Model file for the job. Use its own axes, mm. A direction names the side the tool comes from. Round coordinates to 2 decimals unless told otherwise and drop trailing zeros. Order: outer loops, then holes, each group sorted by start corner. A loop starts at its lowest first (then second) coordinate and runs counter-clockwise, first axis right, second up. Notation, with made-up numbers: (-1.75, 30) - (47.25, 30) arc R28 cw to (47.25, 64) - close; hole circle Ø4 at (27, -29). An arc over 180 degrees is marked (long way). Use one line per item in the form item = value.
from build123d import *

# Parameters (mm, degrees)
BOSS_EXTRUDE3_DEPTH = 59
SKETCH4_W           = 59
SKETCH4_H           = 59
BOSS_EXTRUDE4_DEPTH = 100
SHELL2_T            = -3
SKETCH5_W           = 59
SKETCH5_H           = 59
CUT_EXTRUDE1_DEPTH  = 100
FILLET1_R           = 10


with BuildPart() as part:
    # Sketch3 → Boss-Extrude3 (new body)
    with BuildSketch(Plane.XY):
        with BuildLine():
            Line((-32.434933876, -26.188574195), (26.565066124, -26.188574195))
            Line((26.565066124, -26.188574195), (26.565066124, -36.188574195))
            ThreePointArc((26.565066124, -36.188574195), (33.887396594, -53.866243725), (51.565066124, -61.188574195))
            Line((51.565066124, -61.188574195), (61.565066124, -61.188574195))
            Line((61.565066124, -61.188574195), (61.565066124, -120.188574195))
            Line((61.565066124, -120.188574195), (51.565066124, -120.188574195))
            ThreePointArc((51.565066124, -120.188574195), (-7.831903496, -95.585543815), (-32.434933876, -36.188574195))
            Line((-32.434933876, -36.188574195), (-32.434933876, -26.188574195))
        make_face()
    extrude(amount=BOSS_EXTRUDE3_DEPTH)

    # Sketch4 → Boss-Extrude4 (add)
    with BuildSketch(Plane(origin=(61.565066124, 0, 0), x_dir=(0, 0, -1), z_dir=(1, 0, 0))):
        with Locations((-29.5, -90.688574195)):
            Rectangle(SKETCH4_W, SKETCH4_H)
    extrude(amount=BOSS_EXTRUDE4_DEPTH)

    # Shell2
    shell2_openings = [part.faces().sort_by_distance(p)[0] for p in [
        (-2.934933876, -26.188574195, 29.5),
    ]]
    offset(amount=SHELL2_T, openings=shell2_openings, kind=Kind.INTERSECTION)

    # Sketch5 → Cut-Extrude1 (cut)
    with BuildSketch(Plane(origin=(161.565066124, 0, 0), x_dir=(0, 0, -1), z_dir=(1, 0, 0))):
        with Locations((-29.5, -90.688574195)):
            Rectangle(SKETCH5_W, SKETCH5_H)
    extrude(amount=-CUT_EXTRUDE1_DEPTH, mode=Mode.SUBTRACT)

    # Fillet1
    fillet1_edges = [part.edges().sort_by_distance(p)[0] for p in [
        (56.565066124, -120.188574195, 0),
        (-7.831903496, -95.585543815, 0),
        (-32.434933876, -31.188574195, 0),
        (56.565066124, -120.188574195, 59),
        (33.887396594, -53.866243725, 59),
        (26.565066124, -31.188574195, 59),
        (-29.434933876, -31.188574195, 3),
        (-5.710583152, -93.464223471, 3),
        (56.565066124, -117.188574195, 3),
        (31.76607625, -55.987564069, 3),
        (23.565066124, -31.188574195, 3),
        (-29.434933876, -31.188574195, 56),
        (-5.710583152, -93.464223471, 56),
        (56.565066124, -117.188574195, 56),
        (31.76607625, -55.987564069, 56),
        (23.565066124, -31.188574195, 56),
        (-32.434933876, -31.188574195, 59),
        (56.565066124, -64.188574195, 3),
        (56.565066124, -64.188574195, 56),
        (56.565066124, -61.188574195, 0),
        (56.565066124, -61.188574195, 59),
        (-7.831903496, -95.585543815, 59),
        (26.565066124, -31.188574195, 0),
        (33.887396594, -53.866243725, 0),
    ]]
    fillet(fillet1_edges, radius=FILLET1_R)


solid = part.part
(1) Pin check, flat tips, straight feed: pin 1 (4 mm diameter, centred on y = -105.5, z = 39.5, fed in from +X); pin 2 (3 mm diameter, centred on x = 55, z = 33, fed in from +Y); pin 3 (8 mm diameter, centred on x = -9, z = 23.5, fed in from -Y). Stop position of each tip, or through.
Report:
pin_1 = 13.15
pin_2 = -61.19
pin_3 = -98.29
(2) Pull direction Y, two halves, no side cores. Call faces 1 (the face through (56.64, -114.34, 52.99)), 2 (the face through (-7.175, -96.235, 29.227)), 3 (the face through (20.558, -31.119, 53.148)): released by +Y, released by -Y, zero draft, split by the parting line, or undercut.
Report:
face_1 = undercut
face_2 = released by -Y
face_3 = zero draft
(3) Tool access for faces 4 (the face through (23.565, -31, 29)), 5 (the face through (56.5, -67.2, 53.15)), 6 (the face through (20, -67, 3)): list every direction of +Z, -Z, +X, -X, +Y, -Y with a clear straight run to the whole face (end or side of a thin tool).
Report:
face_4 = +Y
face_5 = +X
face_6 = none
(4) Slice it at B-B on z = 7.5. Give the cut face in (x, y), then the cut area to 3 significant figures.
Report:
outline = (-32.12, -36.19) arc R83.68 ccw to (51.57, -119.87) - (61.57, -119.87) - (61.57, -115.54) - (51.57, -115.54) arc R79.35 cw to (-27.79, -36.19) - (-27.79, -26.19) - (-32.12, -26.19) - close; (21.92, -36.19) arc R29.65 ccw to (51.57, -65.84) - (61.57, -65.84) - (61.57, -61.51) - (51.57, -61.51) arc R25.32 cw to (26.25, -36.19) - (26.25, -26.19) - (21.92, -26.19) - close
area = 915 mm2
(5) Slice it at A-A on z = 32.5. Give the cut face in (x, y), then the cut area to 3 significant figures.
Report:
outline = (-32.43, -36.19) arc R84 ccw to (51.57, -120.19) - (61.57, -120.19) - (61.57, -117.19) - (51.57, -117.19) arc R81 cw to (-29.43, -36.19) - (-29.43, -26.19) - (-32.43, -26.19) - close; (23.57, -36.19) arc R28 ccw to (51.57, -64.19) - (61.57, -64.19) - (61.57, -61.19) - (51.57, -61.19) arc R25 cw to (26.57, -36.19) - (26.57, -26.19) - (23.57, -26.19) - close
area = 634 mm2
(6) Probe probe 1 along Z at (x, y) = (9, -70); probe 2 along Y at (x, z) = (55, 24.5); probe 3 along X at (y, z) = (-30.5, 24.5). List the from-to ranges inside material, lowest first. Write a range as [from, to].
Report:
probe_1 = [0, 3], [56, 59]
probe_2 = [-120.19, -117.19], [-64.19, -61.19]
probe_3 = [-32.43, -29.43], [23.57, 26.57]
